For this review, take the finished solid that the model builds, in its own axes (mm). A direction names the side the tool comes from. Coordinates: 2 decimals unless noted, no trailing zeros. Loops run counter-clockwise (first coordinate to the right, second up) from the corner with the lowest first, then second, coordinate; pieces in that order, holes last. Notation, with made-up numbers: (-4.75, 72.5) - (41.25, 72.5) arc R34 ccw to (41.25, 105.5) - close; hole circle Ø11 at (63, 44). An arc over 180 degrees is marked (long way). Answer as a JSON object with one key per item and string values. Group by question number.
Item 1: Tool access review of faces 4 (the flat face through (0, 0, -36)), 5 (the flat face through (7, 0, 0)), 6 (the cylindrical face through (-6.147, 6.217, -81.338)): name each direction out of +Z, -Z, +X, -X, +Y, -Y from which nothing blocks a thin tool from reaching the whole face with its end or side.
Item 2: We need section C-C (x = 0). Give the boundary of the cut face in (y, z).
Item 3: Mouldability with a two-part tool opening along Z and no side actions: class faces 1 (the cylindrical face through (-5.134, 0.751, 7.385)), 2 (the cylindrical face through (6.217, 6.147, -81.338)), 3 (the flat face through (0, 0, 10)) as released by +Z, released by -Z, zero draft, split by the parting line, or undercut.
Item 4: We need section A-A (y = 0). Give the boundary of the cut face in (x, z), then the cut area to 3 significant figures.
Item 5: Clearance check with flat-ended pins moving along their axes: pin 1 (2 mm diameter, centred on y = -5.5, z = -67.5, fed in from -X); pin 2 (4.5 mm diameter, centred on y = 0, z = -79.5, fed in from -X); pin 3 (8 mm diameter, centred on x = 4, z = -45.5, fed in from +Y). State where each tip first meets the part, or that it passes through.
Item 6: We need section D-D (z = 5). Give the boundary of the cut face in (x, y).
Item 7: We need section B-B (z = -79.5). Give the boundary of the cut face in (x, y), then the cut area to 3 significant figures.
Item 8: To check wall thickness, follow line 1 (Z direction, x = -3.75, y = 0.75); line 2 (Y direction, x = 0, z = -54); line 3 (Z direction, x = 6.75, y = -0.5). State the ranges of each line that lie inside material, in increasing order.
from build123d import *

# Parameters (mm, degrees)
SKETCH_1_W          = 15
SKETCH_1_H          = 15
EXTRUDE_1_DEPTH     = 10
FILLET_1_R          = 4.5
SKETCH_2_R          = 2.5
CUT_EXTRUDE_1_DEPTH = 4.8
SKETCH_4_R          = 6.5
EXTRUDE_2_DEPTH     = 75
SKETCH_6_W          = 15
SKETCH_6_H          = 15
EXTRUDE_3_DEPTH     = 12.5
FILLET_2_R          = 4.5
SKETCH_7_R          = 4.5
EXTRUDE_4_DEPTH     = 8.5
SKETCH_13_R         = 2.5
CUT_EXTRUDE_2_DEPTH = 4.8
SKETCH_16_R         = 2.5
CUT_EXTRUDE_6_DEPTH = 60


with BuildPart() as part:
    # 草图1 → 凸台-拉伸1 (new body)
    with BuildSketch(Plane.XY):
        Rectangle(SKETCH_1_W, SKETCH_1_H)
    extrude(amount=EXTRUDE_1_DEPTH)

    # 圆角1
    fillet_1_edges = [part.edges().sort_by_distance(p)[0] for p in [
        (7.5, -7.5, 5),
        (-7.5, -7.5, 5),
        (-7.5, 7.5, 5),
        (7.5, 7.5, 5),
    ]]
    fillet(fillet_1_edges, radius=FILLET_1_R)

    # 草图2 → 切除-拉伸1 (cut)
    with BuildSketch(Plane.ZY.offset(7.5)):
        with Locations((5, 0)):
            Circle(SKETCH_2_R)
    extrude(amount=-CUT_EXTRUDE_1_DEPTH, mode=Mode.SUBTRACT)

    # 草图4 → 凸台-拉伸2 (add)
    with BuildSketch(Plane(origin=(0, 0, 0), x_dir=(-1, 0, 0), z_dir=(0, 0, -1))):
        Circle(SKETCH_4_R)
    extrude(amount=EXTRUDE_2_DEPTH)

    # 草图6 → 凸台-拉伸3 (add)
    with BuildSketch(Plane(origin=(0, 0, -75), x_dir=(-1, 0, 0), z_dir=(0, 0, -1))):
        Rectangle(SKETCH_6_W, SKETCH_6_H)
    extrude(amount=EXTRUDE_3_DEPTH)

    # 圆角2
    fillet_2_edges = [part.edges().sort_by_distance(p)[0] for p in [
        (-7.5, -7.5, -81.25),
        (-7.5, 7.5, -81.25),
        (7.5, 7.5, -81.25),
        (7.5, -7.5, -81.25),
    ]]
    fillet(fillet_2_edges, radius=FILLET_2_R)

    # 草图7 → 凸台-拉伸4 (add)
    with BuildSketch(Plane(origin=(0, 0, -87.5), x_dir=(-1, 0, 0), z_dir=(0, 0, -1))):
        Circle(SKETCH_7_R)
    extrude(amount=EXTRUDE_4_DEPTH)

    # 草图13 → 切除-拉伸2 (cut)
    with BuildSketch(Plane.ZY.offset(7.5)):
        with Locations((-79.5, 0)):
            Circle(SKETCH_13_R)
    extrude(amount=-CUT_EXTRUDE_2_DEPTH, mode=Mode.SUBTRACT)

    # 草图16 → 切除-拉伸6 (cut)
    with BuildSketch(Plane(origin=(0, 0, -96), x_dir=(-1, 0, 0), z_dir=(0, 0, -1))):
        Circle(SKETCH_16_R)
    extrude(amount=-CUT_EXTRUDE_6_DEPTH, mode=Mode.SUBTRACT)


solid = part.part
Check sheet entries:
{
 "1": {"face 4": "-Z", "face 5": "none", "face 6": "+Z, -Z, -X, +Y"},
 "2": {"outline": "(-7.5, -87.5) - (-4.5, -87.5) - (-4.5, -96) - (-2.5, -96) - (-2.5, -36) - (2.5, -36) - (2.5, -96) - (4.5, -96) - (4.5, -87.5) - (7.5, -87.5) - (7.5, -75) - (6.5, -75) - (6.5, 0) - (7.5, 0) - (7.5, 10) - (-7.5, 10) - (-7.5, 0) - (-6.5, 0) - (-6.5, -75) - (-7.5, -75) - close"},
 "3": {"face 1": "undercut", "face 2": "zero draft", "face 3": "released by +Z"},
 "4": {"outline": "(-7.5, -87.5) - (-4.5, -87.5) - (-4.5, -96) - (-2.5, -96) - (-2.5, -36) - (2.5, -36) - (2.5, -96) - (4.5, -96) - (4.5, -87.5) - (7.5, -87.5) - (7.5, -75) - (6.5, -75) - (6.5, 0) - (7.5, 0) - (7.5, 10) - (-7.5, 10) - (-7.5, 7.5) - (-2.7, 7.5) - (-2.7, 2.5) - (-7.5, 2.5) - (-7.5, 0) - (-6.5, 0) - (-6.5, -75) - (-7.5, -75) - (-7.5, -77) - (-2.7, -77) - (-2.7, -82) - (-7.5, -82) - close", "area": "1,040 mm2"},
 "5": {"pin 1": "stops at x = -4.69", "pin 2": "stops at x = -2.7", "pin 3": "stops at y = 6.5"},
 "6": {"outline": "(-7.5, -3) arc R4.5 ccw to (-3, -7.5) - (3, -7.5) arc R4.5 ccw to (7.5, -3) - (7.5, 3) arc R4.5 ccw to (3, 7.5) - (-3, 7.5) arc R4.5 ccw to (-7.5, 3) - (-7.5, 2.5) - (-2.7, 2.5) - (-2.7, -2.5) - (-7.5, -2.5) - close"},
 "7": {"outline": "(-7.5, -3) arc R4.5 ccw to (-3, -7.5) - (3, -7.5) arc R4.5 ccw to (7.5, -3) - (7.5, 3) arc R4.5 ccw to (3, 7.5) - (-3, 7.5) arc R4.5 ccw to (-7.5, 3) - (-7.5, 2.5) - (-2.7, 2.5) - (-2.7, -2.5) - (-7.5, -2.5) - close; hole circle Ø5 at (0, 0)", "area": "164 mm2"},
 "8": {"line 1": "z = -96 to -81.88, -77.12 to 2.62, 7.38 to 10", "line 2": "y = -6.5 to -2.5, 2.5 to 6.5", "line 3": "z = -87.5 to -75, 0 to 10"}
}
